Print and shaded views of the part. All mm, measured from the part's lowest x, y and z. Coordinates: 2 decimals unless noted, no trailing zeros. Order: outer loops, then holes, each group sorted by start corner. A loop starts at its lowest first (then second) coordinate and runs counter-clockwise, first axis right, second up. Notation, with made-up numbers: (-31.5, 79) -> (-7.5, 79) arc R36 ccw to (-7.5, 117) -> close; hole circle Ø4 at (71.25, 74.25). An arc over 180 degrees is marked (long way). Return JSON: item names as keys, results as strings. Group by question number.
1) Cut at D-D (z = 285). Write the cut outline in (x, y), and give its area (3 significant figures).
2) Flat gauge pins, fed straight in: pin 1 (3 mm diameter, centred on x = 5, y = 399.5, fed in from -Z); pin 2 (5 mm diameter, centred on x = 3, z = 107, fed in from +Y); pin 3 (3 mm diameter, centred on x = 6.5, y = 585, fed in from +Z). Where does each tip first touch, or does it go through?
3) Cut at C-C (x = 3.5). Write the cut outline in (y, z), and give its area (3 significant figures).
4) Cut at A-A (z = 356.5). Write the cut outline in (x, y), and give its area (3 significant figures).
5) Probe line 1 (Y direction, x = 6.25, z = 238); line 2 (Y direction, x = 3.5, z = 190.5); line 3 (Z direction, x = 5.5, y = 860). List the from-to ranges inside material, lowest first.
6) Cut at B-B (y = 813). Write the cut outline in (x, z), and give its area (3 significant figures).
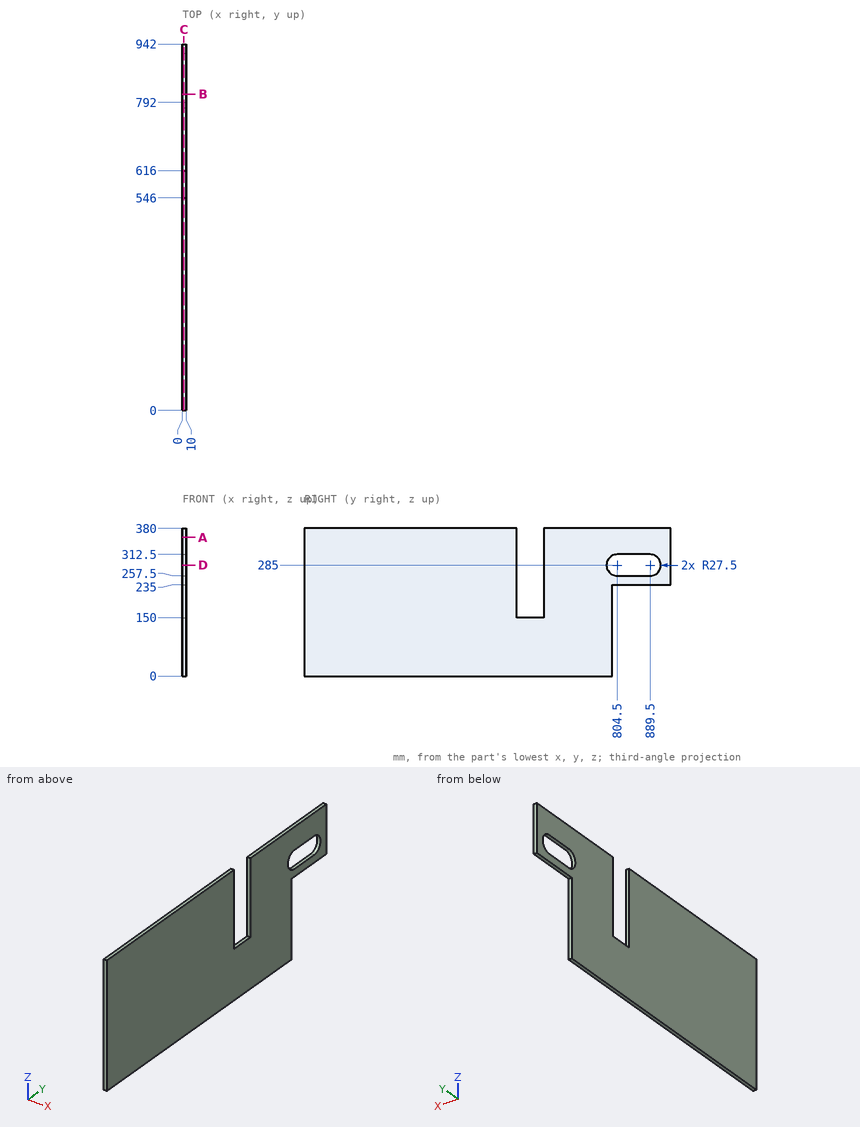
Answers below:
{
 "1": {"outline": "(0, 0) -> (10, 0) -> (10, 546) -> (0, 546) -> close; (0, 616) -> (10, 616) -> (10, 777) -> (0, 777) -> close; (0, 917) -> (10, 917) -> (10, 942) -> (0, 942) -> close", "area": "7,320 mm^2"},
 "2": {"pin 1": "stops at z = 0", "pin 2": "stops at y = 792", "pin 3": "stops at z = 150"},
 "3": {"outline": "(0, 0) -> (792, 0) -> (792, 235) -> (942, 235) -> (942, 380) -> (616, 380) -> (616, 150) -> (546, 150) -> (546, 380) -> (0, 380) -> close; hole (804.5, 257.5) -> (889.5, 257.5) arc R27.5 ccw to (889.5, 312.5) -> (804.5, 312.5) arc R27.5 ccw to start", "area": "300,000 mm^2"},
 "4": {"outline": "(0, 0) -> (10, 0) -> (10, 546) -> (0, 546) -> close; (0, 616) -> (10, 616) -> (10, 942) -> (0, 942) -> close", "area": "8,720 mm^2"},
 "5": {"line 1": "y = 0 to 546, 616 to 942", "line 2": "y = 0 to 546, 616 to 792", "line 3": "z = 235 to 257.5, 312.5 to 380"},
 "6": {"outline": "(0, 235) -> (10, 235) -> (10, 257.5) -> (0, 257.5) -> close; (0, 312.5) -> (10, 312.5) -> (10, 380) -> (0, 380) -> close", "area": "900 mm^2"}
}
